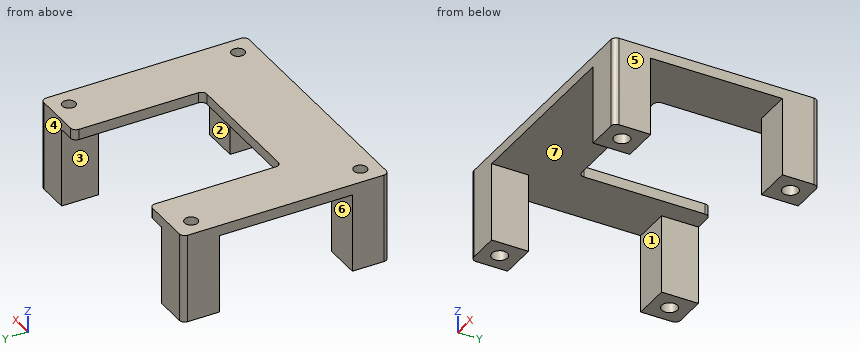
```python
from build123d import *

# Parameters (mm, degrees)
SKETCH_R     = 1.25
PAD_DEPTH    = 2
SKETCH001_W  = 7
SKETCH001_H  = 7
SKETCH001_R  = 1.5
PAD001_DEPTH = 15
FILLET_R     = 1
FILLET001_R  = 1
FILLET002_R  = 1
FILLET003_R  = 1
FILLET004_R  = 1
FILLET005_R  = 1
FILLET006_R  = 1
FILLET007_R  = 1


with BuildPart() as part:
    # Sketch → Pad (new body)
    with BuildSketch(Plane.XY):
        Polygon((24, 19.364391), (24, -19.635609), (-24, -19.635609), (-24, 19.635609), (-13, 19.635609), (-13, -5.364391), (13, -5.364391), (13, 19.364391), align=None)
        with Locations((-20.5, 16)):
            Circle(SKETCH_R, mode=Mode.SUBTRACT)
        with Locations((20.5, -16.135609)):
            Circle(SKETCH_R, mode=Mode.SUBTRACT)
        with Locations((20.5, 16)):
            Circle(SKETCH_R, mode=Mode.SUBTRACT)
        with Locations((-20.5, -16.135609)):
            Circle(SKETCH_R, mode=Mode.SUBTRACT)
    extrude(amount=PAD_DEPTH)

    # Sketch001 → Pad001 (join)
    with BuildSketch(Plane.XY):
        with Locations((-20.5, 16.135609)):
            Rectangle(SKETCH001_W, SKETCH001_H)
        with Locations((-20.5, 16.135609)):
            Circle(SKETCH001_R, mode=Mode.SUBTRACT)
        with Locations((20.5, 15.864391)):
            Rectangle(SKETCH001_W, SKETCH001_H)
        with Locations((20.5, 15.864391)):
            Circle(SKETCH001_R, mode=Mode.SUBTRACT)
        with Locations((-20.5, -16.135609)):
            Rectangle(SKETCH001_W, SKETCH001_H)
        with Locations((-20.5, -16.135609)):
            Circle(SKETCH001_R, mode=Mode.SUBTRACT)
        with Locations((20.5, -16.135609)):
            Rectangle(SKETCH001_W, SKETCH001_H)
        with Locations((20.5, -16.135609)):
            Circle(SKETCH001_R, mode=Mode.SUBTRACT)
    extrude(amount=-PAD001_DEPTH)

    # Fillet
    fillet_edges = [part.edges().sort_by_distance(p)[0] for p in [
        (24, -19.635609, -7.5),
        (24, -19.635609, 1),
    ]]
    fillet(fillet_edges, radius=FILLET_R)

    # Fillet001
    fillet001_edges = [part.edges().sort_by_distance(p)[0] for p in [
        (24, 19.364391, 1),
        (24, 19.364391, -7.5),
    ]]
    fillet(fillet001_edges, radius=FILLET001_R)

    # Fillet002
    fillet002_edges = [part.edges().sort_by_distance(p)[0] for p in [
        (-24, 19.635609, 1),
        (-24, 19.635609, -7.5),
    ]]
    fillet(fillet002_edges, radius=FILLET002_R)

    # Fillet003
    fillet003_edges = [part.edges().sort_by_distance(p)[0] for p in [
        (-24, -19.635609, -7.5),
        (-24, -19.635609, 1),
    ]]
    fillet(fillet003_edges, radius=FILLET003_R)

    # Fillet004
    fillet004_edges = [part.edges().sort_by_distance(p)[0] for p in [
        (-13, 19.635609, 1),
    ]]
    fillet(fillet004_edges, radius=FILLET004_R)

    # Fillet005
    fillet005_edges = [part.edges().sort_by_distance(p)[0] for p in [
        (-13, -5.364391, 1),
    ]]
    fillet(fillet005_edges, radius=FILLET005_R)

    # Fillet006
    fillet006_edges = [part.edges().sort_by_distance(p)[0] for p in [
        (13, -5.364391, 1),
    ]]
    fillet(fillet006_edges, radius=FILLET006_R)

    # Fillet007
    fillet007_edges = [part.edges().sort_by_distance(p)[0] for p in [
        (13, 19.364391, 1),
    ]]
    fillet(fillet007_edges, radius=FILLET007_R)


solid = part.part
```
Design review of the part built by this model. Coordinates are the model's own, in mm. Face numbers are marked on the shaded views. A direction names the side the tool comes from. Coordinates: 2 decimals unless noted, no trailing zeros. Loops run counter-clockwise (first coordinate to the right, second up) from the corner with the lowest first, then second, coordinate; pieces in that order, holes last. Notation, with made-up numbers: (71, 49) - (99, 49) arc R21 cw to (99, 58) - close; hole circle Ø2 at (-37.5, 59.25). An arc over 180 degrees is marked (long way). Use CSV: the item, a comma, the result in double quotes. Start each with the question number.
1) Consider section C-C on x = 20.5. Write out the cut boundary in (y, z), then the cut area to 3 significant figures.
2) Consider section A-A on y = 6. Write out the cut boundary in (x, z), then the cut area to 3 significant figures.
3) For pin 1 Ø3 at (y, z) = (12, -9) entering from -X; pin 2 Ø0.6 at (x, z) = (1.5, 1) entering from +Y; pin 3 Ø5 at (x, y) = (-12.5, 15.5) entering from -Z, all flat-tipped, find the tip position at first contact; note any pin that passes through.
4) Consider section B-B on z = -6. Write out the cut boundary in (x, y).
5) The part is to be moulded in two halves that separate along X. For the marked faces 5, 6 and 7, say which applies: +X half, -X half, draft (parallel to the pull), parting line (faces both ways), or undercut.
6) Wall thickness on L1, parallel to Y at x = 20.5, z = 1.05; L2, parallel to X at y = 16, z = -7.5; L3, parallel to Y at x = 20.5, z = -5.75: over which ranges is each line inside the solid? List them lowest first. Write a range as from..to.
7) Consider section D-D on x = -20.5. Write out the cut boundary in (y, z).
8) Tool access review of the marked faces 1, 2, 3 and 4: name each direction out of +Z, -Z, +X, -X, +Y, -Y from which nothing blocks a thin tool from reaching the whole face with its end or side.
Geometry says:
1,outline,"(-19.64, -15) - (-17.64, -15) - (-17.64, 0) - (-17.39, 0) - (-17.39, 2) - (-19.64, 2) - close; (-14.89, 0) - (-14.64, 0) - (-14.64, -15) - (-12.64, -15) - (-12.64, 0) - (12.36, 0) - (12.36, -15) - (14.36, -15) - (14.36, 0) - (14.75, 0) - (14.75, 2) - (-14.89, 2) - close; (17.25, 0) - (17.36, 0) - (17.36, -15) - (19.36, -15) - (19.36, 2) - (17.25, 2) - close"
1,area,"188 mm^2"
2,outline,"(-24, 0) - (-13, 0) - (-13, 2) - (-24, 2) - close; (13, 0) - (24, 0) - (24, 2) - (13, 2) - close"
2,area,"44.0 mm^2"
3,pin 1,"x = -24"
3,pin 2,"y = -5.36"
3,pin 3,"z = 0"
4,outline,"(-24, -18.64) arc R1 ccw to (-23, -19.64) - (-17, -19.64) - (-17, -12.64) - (-24, -12.64) - close; (-24, 12.64) - (-17, 12.64) - (-17, 19.64) - (-23, 19.64) arc R1 ccw to (-24, 18.64) - close; (17, -19.64) - (23, -19.64) arc R1 ccw to (24, -18.64) - (24, -12.64) - (17, -12.64) - close; (17, 12.36) - (24, 12.36) - (24, 18.36) arc R1 ccw to (23, 19.36) - (17, 19.36) - close; hole circle Ø3 at (-20.5, -16.14); hole circle Ø3 at (-20.5, 16.14); hole circle Ø3 at (20.5, -16.14); hole circle Ø3 at (20.5, 15.86)"
5,face 5,"+X half"
5,face 6,"draft"
5,face 7,"undercut"
6,L1,"-19.64..-17.39, -14.89..14.75, 17.25..19.36"
6,L2,"-24..-21.99, -19.01..-17, 17..19.01, 21.99..24"
6,L3,"-19.64..-17.64, -14.64..-12.64, 12.36..14.36, 17.36..19.36"
7,outline,"(-19.64, -15) - (-17.64, -15) - (-17.64, 0) - (-17.39, 0) - (-17.39, 2) - (-19.64, 2) - close; (-14.89, 0) - (-14.64, 0) - (-14.64, -15) - (-12.64, -15) - (-12.64, 0) - (12.64, 0) - (12.64, -15) - (14.64, -15) - (14.64, 0) - (14.75, 0) - (14.75, 2) - (-14.89, 2) - close; (17.25, 0) - (17.64, 0) - (17.64, -15) - (19.64, -15) - (19.64, 2) - (17.25, 2) - close"
8,face 1,"-Z, -X"
8,face 2,"-Z, +X, -X"
8,face 3,"-Z, +Y, -Y"
8,face 4,"+Z, -Z, +X, +Y"
